The model under review builds one solid part; all positions refer to its coordinate system, in mm. A direction names the side the tool comes from. Give positions to 0.01 mm unless a question says otherwise; leave off trailing zeros. Order: outer loops, then holes, each group sorted by start corner. A loop starts at its lowest first (then second) coordinate and runs counter-clockwise, first axis right, second up.
```python
from build123d import *

# Parameters (mm, degrees)
SKETCH1_W                 = 17.78
SKETCH1_H                 = 74.93
BOSS_EXTRUDE1_DEPTH       = 12.7
CUT_EXTRUDE1_DEPTH        = 10.16
TAP_DRILL_FOR_6_32_TAP1_D = 2.7051
SKETCH5_R                 = 2.39395
CUT_EXTRUDE2_DEPTH        = 11.1125


with BuildPart() as part:
    # Sketch1 → Boss-Extrude1 (new body)
    with BuildSketch(Plane(origin=(0, 0, 0), x_dir=(0, 0, -1), z_dir=(1, 0, 0))):
        with Locations((8.89, 37.465)):
            Rectangle(SKETCH1_W, SKETCH1_H)
    extrude(amount=BOSS_EXTRUDE1_DEPTH)

    # Sketch2 → Cut-Extrude1 (cut)
    with BuildSketch(Plane(origin=(12.7, 0, 0), x_dir=(0, 0, -1), z_dir=(1, 0, 0))):
        Polygon((0, 64.77), (10.16, 64.77), (13.97, 64.77), (24.13, 64.77), (24.13, 10.16), (13.97, 10.16), (10.16, 10.16), (0, 10.16), align=None)
    extrude(amount=-CUT_EXTRUDE1_DEPTH, mode=Mode.SUBTRACT)

    # Tap Drill for #6-32 Tap1 (through all)
    with Locations(Plane(origin=(12.7, 0, 0), x_dir=(0, 0, -1), z_dir=(1, 0, 0))):
        with Locations((5.08, 69.85), (5.08, 5.08)):
            Hole(TAP_DRILL_FOR_6_32_TAP1_D / 2)

    # Sketch5 → Cut-Extrude2 (cut)
    with BuildSketch(Plane(origin=(0, 0, -17.78), x_dir=(-1, 0, 0), z_dir=(0, 0, -1))):
        with Locations((-6.35, 69.85)):
            Circle(SKETCH5_R)
        with BuildLine():
            Line((-8.74395, 4.953), (-8.74395, 5.207))
            ThreePointArc((-8.74395, 5.207), (-6.35, 7.60095), (-3.95605, 5.207))
            Line((-3.95605, 5.207), (-3.95605, 4.953))
            ThreePointArc((-3.95605, 4.953), (-6.35, 2.55905), (-8.74395, 4.953))
        make_face()
    extrude(amount=-CUT_EXTRUDE2_DEPTH, mode=Mode.SUBTRACT)


solid = part.part
```
Item 1: Take a section at B-B (z = -9). Give the boundary of the cut face in (x, y), and give its area (3 significant figures).
Values found:
outline: (0, 0) - (12.7, 0) - (12.7, 10.16) - (2.54, 10.16) - (2.54, 64.77) - (12.7, 64.77) - (12.7, 74.93) - (0, 74.93) - close; hole (3.96, 4.95) arc R2.39 ccw to (8.74, 4.95) - (8.74, 5.21) arc R2.39 ccw to (3.96, 5.21) - close; hole circle Ø4.79 at (6.35, 69.85)
area: 360 mm2
Item 2: Take a section at D-D (z = -5.08). Give the boundary of the cut face in (x, y).
Values found:
outline: (0, 0) - (12.7, 0) - (12.7, 3.73) - (0, 3.73) - close; (0, 6.43) - (12.7, 6.43) - (12.7, 10.16) - (2.54, 10.16) - (2.54, 64.77) - (12.7, 64.77) - (12.7, 68.5) - (0, 68.5) - close; (0, 71.2) - (12.7, 71.2) - (12.7, 74.93) - (0, 74.93) - close
Item 3: Take a section at C-C (y = 69.85). Give the boundary of the cut face in (x, z), and give its area (3 significant figures).
Values found:
outline: (0, -17.78) - (3.96, -17.78) - (3.96, -6.67) - (8.74, -6.67) - (8.74, -17.78) - (12.7, -17.78) - (12.7, -6.43) - (0, -6.43) - close; (0, -3.73) - (12.7, -3.73) - (12.7, 0) - (0, 0) - close
area: 138 mm2
Item 4: Clearance check with flat-ended pins moving along their axes: pin 1 Ø3 at (x, y) = (2, 43.5) entering from +Z; pin 2 Ø1.5 at (y, z) = (44.5, -15.5) entering from +X. State where each tip first meets the part, or that it passes through.
Values found:
pin 1: stops at z = 0
pin 2: stops at x = 2.54
Item 5: For faces 5 (the flat face through (6, 0, -9)), 6 (the flat face through (8, 10.16, -9)), 7 (the cylindrical face through (6.3, 2.56, -12.3)), list the 3-axis set-ups (+Z, -Z, +X, -X, +Y, -Y) from which the entire face can be reached by the end or side of a thin tool; tool diameter is ignored.
Values found:
face 5: +Z, -Z, +X, -X, -Y
face 6: +Z, -Z, +X
face 7: -Z
Item 6: Draft analysis for pull direction X (two halves, no side actions). For faces 1 (the flat face through (12.7, 70, -9)), 2 (the flat face through (6, 5, -6.668)), 3 (the flat face through (6, 70, -6.668)), 4 (the cylindrical face through (6.26, 71.19, -5.26)), state which applies: released by +X, released by -X, zero draft, split by the parting line, or undercut.
Values found:
face 1: released by +X
face 2: undercut
face 3: undercut
face 4: zero draft
Item 7: Take a section at A-A (x = 3.25). Give the boundary of the cut face in (y, z).
Values found:
outline: (0, -17.78) - (10.16, -17.78) - (10.16, 0) - (0, 0) - close; (64.77, -17.78) - (74.93, -17.78) - (74.93, 0) - (64.77, 0) - close; hole circle Ø2.71 at (5.08, -5.08); hole circle Ø2.71 at (69.85, -5.08)
Item 8: For line 1 (Y direction, x = 8.5, z = -5.08); line 2 (Y direction, x = 6.35, z = -15); line 3 (Y direction, x = 11.25, z = -1.25), list the stretches that pass through material, from the lowest coordinate up.
Values found:
line 1: y = 0 to 3.73, 6.43 to 10.16, 64.77 to 68.5, 71.2 to 74.93
line 2: y = 0 to 2.56, 7.6 to 10.16, 64.77 to 67.46, 72.24 to 74.93
line 3: y = 0 to 10.16, 64.77 to 74.93
